Work out the finished part from the listing and answer in its coordinate system (mm). Face numbers are marked on the shaded views. A direction names the side the tool comes from. Coordinates: 2 decimals unless noted, no trailing zeros. Loops run counter-clockwise (first coordinate to the right, second up) from the corner with the lowest first, then second, coordinate; pieces in that order, holes last.
```python
from build123d import *
from build123d.topology import SkipClean

# Parameters (mm, degrees)
ESQUISSE1_W             = 64
ESQUISSE1_H             = 95
ESQUISSE1_R             = 16
BOSS_EXTRU_1_DEPTH      = 12
ESQUISSE2_W             = 48
ESQUISSE2_H             = 95
ENL_V_MAT_EXTRU_1_DEPTH = 2.6
ESQUISSE3_W             = 42
ESQUISSE3_H             = 95
ENL_V_MAT_EXTRU_2_DEPTH = 0.6
ESQUISSE4_R             = 1.6
ENL_V_MAT_EXTRU_4_DEPTH = 78.897368377
ENL_V_MAT_EXTRU_5_DEPTH = 5
CONG_1_R                = 2
BOSS_EXTRU_2_START      = 1
ESQUISSE6_R             = 1.6
BOSS_EXTRU_2_DEPTH      = 1


with BuildPart() as part:
    # Esquisse1 → Boss.-Extru.1 (new body)
    with BuildSketch(Plane.XY):
        with Locations((0, 22.5)):
            Rectangle(ESQUISSE1_W, ESQUISSE1_H)
        Circle(ESQUISSE1_R, mode=Mode.SUBTRACT)
    extrude(amount=-BOSS_EXTRU_1_DEPTH)

    # Esquisse2 → Enlèv. mat.-Extru.1 (cut)
    with BuildSketch(Plane.XY):
        with Locations((0, 22.5)):
            Rectangle(ESQUISSE2_W, ESQUISSE2_H)
    extrude(amount=-ENL_V_MAT_EXTRU_1_DEPTH, mode=Mode.SUBTRACT)

    # Esquisse3 → Enlèv. mat.-Extru.2 (cut)
    with BuildSketch(Plane.XY.offset(-2.6)):
        with Locations((0, 22.5)):
            Rectangle(ESQUISSE3_W, ESQUISSE3_H)
    extrude(amount=-ENL_V_MAT_EXTRU_2_DEPTH, mode=Mode.SUBTRACT)

    # Esquisse4 → Enlèv. mat.-Extru.4 (cut, through all)
    with BuildSketch(Plane.XY):
        with Locations((-28, -19)):
            Circle(ESQUISSE4_R)
        with Locations((-28, 22.5)):
            Circle(ESQUISSE4_R)
        with Locations((-28, 64)):
            Circle(ESQUISSE4_R)
    enl_v_mat_extru_4 = extrude(amount=-ENL_V_MAT_EXTRU_4_DEPTH, mode=Mode.SUBTRACT)

    # Symétrie1: Enlèv. mat.-Extru.4 across plane
    add(enl_v_mat_extru_4.mirror(Plane(origin=(0, 0, 0), x_dir=(0, 0, 1), z_dir=(1, 0, 0))), mode=Mode.SUBTRACT)

    # Esquisse5 → Enlèv. mat.-Extru.5 (cut)
    with BuildSketch(Plane.XY.offset(-3.2)):
        with BuildLine():
            Line((16, 70), (9.817340904, 38.097418184))
            ThreePointArc((9.817340904, 38.097418184), (0, 30), (-9.817340904, 38.097418184))
            Line((-9.817340904, 38.097418184), (-16, 70))
            Line((-16, 70), (16, 70))
        make_face()
    extrude(amount=-ENL_V_MAT_EXTRU_5_DEPTH, mode=Mode.SUBTRACT)

    # Congé1
    cong_1_edges = [part.edges().sort_by_distance(p)[0] for p in [
        (-32, 70, -6),
        (32, 70, -6),
        (32, -25, -6),
        (-32, -25, -6),
        (-16, 70, -5.7),
        (16, 70, -5.7),
    ]]
    fillet(cong_1_edges, radius=CONG_1_R)

    # Esquisse6 → Boss.-Extru.2 (add)
    # profile 1 of 2: a face of its own
    with SkipClean():  # the faces are left unmerged after this step: merging them gives an invalid solid
        with BuildSketch(Plane.XY.offset(BOSS_EXTRU_2_START)):
            with BuildLine():
                Line((-32, 68), (-32, -23))
                ThreePointArc((-32, -23), (-31.414213562, -24.414213562), (-30, -25))
                Line((-30, -25), (-24, -25))
                Line((-24, -25), (-24, 70))
                Line((-24, 70), (-30, 70))
                ThreePointArc((-30, 70), (-31.414213562, 69.414213562), (-32, 68))
            make_face()
            with Locations((-28, 64)):
                Circle(ESQUISSE6_R, mode=Mode.SUBTRACT)
            with Locations((-28, 22.5)):
                Circle(ESQUISSE6_R, mode=Mode.SUBTRACT)
            with Locations((-28, -19)):
                Circle(ESQUISSE6_R, mode=Mode.SUBTRACT)
        # profile 2 of 2: a face of its own
        with BuildSketch(Plane.XY.offset(BOSS_EXTRU_2_START)):
            with BuildLine():
                Line((32, -23), (32, 68))
                ThreePointArc((32, 68), (31.414213562, 69.414213562), (30, 70))
                Line((30, 70), (24, 70))
                Line((24, 70), (24, -25))
                Line((24, -25), (30, -25))
                ThreePointArc((30, -25), (31.414213562, -24.414213562), (32, -23))
            make_face()
            with Locations((28, -19)):
                Circle(ESQUISSE6_R, mode=Mode.SUBTRACT)
            with Locations((28, 22.5)):
                Circle(ESQUISSE6_R, mode=Mode.SUBTRACT)
            with Locations((28, 64)):
                Circle(ESQUISSE6_R, mode=Mode.SUBTRACT)
        extrude(amount=-BOSS_EXTRU_2_DEPTH)


solid = part.part
```
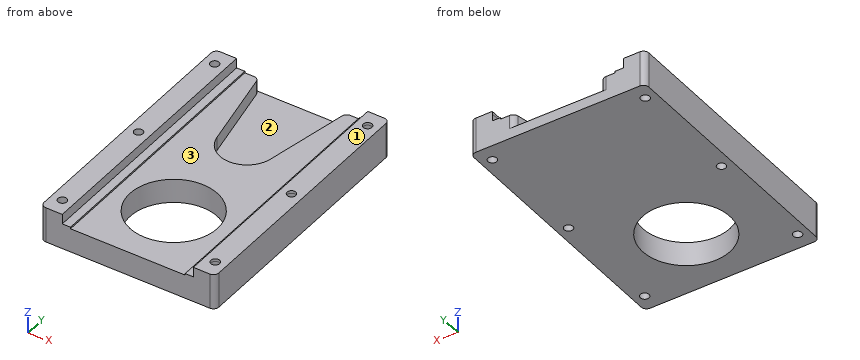
1. A cutting plane is placed at A-A, the plane y = 22.5. Give the vertices of the cut face in (x, z), then the cut area to 3 significant figures.
2. Each of these flat-tipped pins is pushed along its axis until it touches: P1, Ø1.9, axis at x = 28, y = -19, coming from the -Z side; P2, Ø12.5, axis at x = -6.5, y = 18.5, coming from the +Z side; P3, Ø1.5, axis at x = -22.5, y = 45.5, coming from the +Z side. Where does it stop, or does it pass through?
3. A cutting plane is placed at D-D, the plane z = -4.75. Give the vertices of the cut face in (x, y).
4. For the marked faces 1, 2 and 3, determine the directions among +Z, -Z, +X, -X, +Y, -Y from which every point of the face is accessible in a straight line to the end or side of a thin tool.
5. A cutting plane is placed at C-C, the plane y = 0. Give the vertices of the cut face in (x, z).
6. Straight lines are drawn through the part: probe 1 along Y at (x, z) = (-28, -8); probe 2 along X at (y, z) = (36, -1.75); probe 3 along X at (y, z) = (64, -5). For each, find the intervals that lie inside material, in ascending order.
7. A cutting plane is placed at B-B, the plane x = 28. Give the vertices of the cut face in (y, z).
Answers below:
1. outline: (-32, -12) - (-29.6, -12) - (-29.6, 1) - (-32, 1) - close; (-26.4, -12) - (26.4, -12) - (26.4, 1) - (24, 1) - (24, -2.6) - (21, -2.6) - (21, -3.2) - (-21, -3.2) - (-21, -2.6) - (-24, -2.6) - (-24, 1) - (-26.4, 1) - close; (29.6, -12) - (32, -12) - (32, 1) - (29.6, 1) - close
1. area: 551 mm2
2. P1: passes through
2. P2: stops at z = -3.2
2. P3: stops at z = -2.6
3. outline: (-32, -23) arc R2 ccw to (-30, -25) - (30, -25) arc R2 ccw to (32, -23) - (32, 68) arc R2 ccw to (30, 70) - (17.65, 70) arc R2 ccw to (15.69, 68.38) - (9.82, 38.1) arc R10 cw to (-9.82, 38.1) - (-15.69, 68.38) arc R2 ccw to (-17.65, 70) - (-30, 70) arc R2 ccw to (-32, 68) - close; hole circle Ø3.2 at (-28, -19); hole circle Ø3.2 at (-28, 22.5); hole circle Ø3.2 at (-28, 64); hole circle Ø32 at (0, 0); hole circle Ø3.2 at (28, -19); hole circle Ø3.2 at (28, 22.5); hole circle Ø3.2 at (28, 64)
4. face 1: +Z, +X, -X, +Y, -Y
4. face 2: +Z, +Y
4. face 3: +Z, +Y, -Y
5. outline: (-32, -12) - (-16, -12) - (-16, -3.2) - (-21, -3.2) - (-21, -2.6) - (-24, -2.6) - (-24, 1) - (-32, 1) - close; (16, -12) - (32, -12) - (32, 1) - (24, 1) - (24, -2.6) - (21, -2.6) - (21, -3.2) - (16, -3.2) - close
6. probe 1: y = -25 to -20.6, -17.4 to 20.9, 24.1 to 62.4, 65.6 to 70
6. probe 2: x = -32 to -24, 24 to 32
6. probe 3: x = -32 to -29.6, -26.4 to -14.84, 14.84 to 26.4, 29.6 to 32
7. outline: (-25, -12) - (-20.6, -12) - (-20.6, 1) - (-25, 1) - close; (-17.4, -12) - (20.9, -12) - (20.9, 1) - (-17.4, 1) - close; (24.1, -12) - (62.4, -12) - (62.4, 1) - (24.1, 1) - close; (65.6, -12) - (70, -12) - (70, 1) - (65.6, 1) - close
